from build123d import *

# Parameters (mm, degrees)
SKETCH_1_W          = 90
SKETCH_1_H          = 48
EXTRUDE_1_DEPTH     = 40
CUT_EXTRUDE_1_DEPTH = 40
CUT_EXTRUDE_2_DEPTH = 110.562767398
CUT_EXTRUDE_3_DEPTH = 110.562767398
CUT_EXTRUDE_4_DEPTH = 33
SKETCH_6_W          = 8
SKETCH_6_H          = 40
CUT_EXTRUDE_5_DEPTH = 110.562767398
SKETCH_7_W          = 20
SKETCH_7_H          = 13.155555556
CUT_EXTRUDE_6_DEPTH = 5
SKETCH_8_W          = 28.2
SKETCH_8_H          = 28
EXTRUDE_2_DEPTH     = 3
SKETCH_9_R          = 2.25
EXTRUDE_3_DEPTH     = 4
SKETCH_10_R         = 1.2
CUT_EXTRUDE_7_DEPTH = 104.889364229
FILLET_1_R          = 5
FILLET_2_R          = 2.5


with BuildPart() as part:
    # 스케치1 → 보스-돌출1 (new body)
    with BuildSketch(Plane(origin=(0, 0, 0), x_dir=(0, 0, -1), z_dir=(1, 0, 0))):
        with Locations((45, 24)):
            Rectangle(SKETCH_1_W, SKETCH_1_H)
    extrude(amount=EXTRUDE_1_DEPTH)

    # 스케치2 → 컷-돌출1 (cut)
    with BuildSketch(Plane(origin=(40, 0, 0), x_dir=(0, 0, -1), z_dir=(1, 0, 0))):
        Polygon((79, 44), (83, 44), (83, 38), (85.598076211, 36.5), (83, 35), (83, 33.5), (90, 33.5), (90, 14.5), (83, 14.5), (83, 13), (85.598076211, 11.5), (83, 10), (83, 4), (79, 4), align=None)
        Polygon((0, 38), (63.304035288, 48), (0, 48), align=None)
        Polygon((0, 10), (63.304035288, 0), (0, 0), align=None)
    extrude(amount=-CUT_EXTRUDE_1_DEPTH, mode=Mode.SUBTRACT)

    # 스케치3 → 컷-돌출2 (cut, through all)
    with BuildSketch(Plane(origin=(0, 48, 0), x_dir=(1, 0, 0), z_dir=(0, 1, 0))):
        Polygon((0, 67.846768337), (20, 79), (20, 90), (0, 90), align=None)
    extrude(amount=-CUT_EXTRUDE_2_DEPTH, mode=Mode.SUBTRACT)

    # 스케치4 → 컷-돌출3 (cut, through all)
    with BuildSketch(Plane(origin=(0, 48, 0), x_dir=(1, 0, 0), z_dir=(0, 1, 0))):
        Polygon((40, 63.304035288), (14.807552651, 0), (40, 0), align=None)
    extrude(amount=-CUT_EXTRUDE_3_DEPTH, mode=Mode.SUBTRACT)

    # 스케치5 → 컷-돌출4 (cut)
    with BuildSketch(Plane(origin=(40, 0, 0), x_dir=(0, 0, -1), z_dir=(1, 0, 0))):
        Polygon((4.2, 34.488888889), (63.304035288, 34.488888889), (63.304035288, 48), (0, 38), (0, 10), (63.304035288, 0), (63.304035288, 13.511111111), (4.2, 13.511111111), (4.2, 17.422222222), (63.304035288, 17.422222222), (63.304035288, 30.577777778), (4.2, 30.577777778), align=None)
    extrude(amount=-CUT_EXTRUDE_4_DEPTH, mode=Mode.SUBTRACT)

    # 스케치6 → 컷-돌출5 (cut, through all)
    with BuildSketch(Plane(origin=(40, 0, 0), x_dir=(0, 0, -1), z_dir=(1, 0, 0))):
        with Locations((72, 24)):
            Rectangle(SKETCH_6_W, SKETCH_6_H)
    extrude(amount=-CUT_EXTRUDE_5_DEPTH, mode=Mode.SUBTRACT)

    # 스케치7 → 컷-돌출6 (cut)
    with BuildSketch(Plane.XY.offset(-63.304035288)):
        with Locations((30, 24)):
            Rectangle(SKETCH_7_W, SKETCH_7_H)
    extrude(amount=-CUT_EXTRUDE_6_DEPTH, mode=Mode.SUBTRACT)

    # 스케치8 → 보스-돌출2 (add)
    with BuildSketch(Plane.ZY):
        with Locations((-14.1, 24)):
            Rectangle(SKETCH_8_W, SKETCH_8_H)
    extrude(amount=EXTRUDE_2_DEPTH)

    # 스케치9 → 보스-돌출3 (add)
    with BuildSketch(Plane(origin=(0, 0, -79), x_dir=(-1, 0, 0), z_dir=(0, 0, -1))):
        with Locations(Location((-30, 24, 0), (0, 0, 180))):
            Circle(SKETCH_9_R)
    extrude(amount=EXTRUDE_3_DEPTH)

    # 스케치10 → 컷-돌출7 (cut, through all)
    with BuildSketch(Plane(origin=(0, 0, -83), x_dir=(-1, 0, 0), z_dir=(0, 0, -1))):
        with Locations((-30, 24)):
            Circle(SKETCH_10_R)
    extrude(amount=-CUT_EXTRUDE_7_DEPTH, mode=Mode.SUBTRACT)

    # 필렛1
    # the kernel refuses this fillet: 5 mm, written as the material it takes off along each edge
    with BuildSketch(Plane(origin=(-3, 49.456439237, -28.2), x_dir=(1, 0, 0), z_dir=(0, -1, 0))) as fillet_1_piece_1:
        with BuildLine():
            CenterArc((5, 4.582575695), FILLET_1_R, 180, 66.421821522)
            Line((0, 4.582575695), (-0.1, 4.582575695))
            Line((-0.1, 4.582575695), (-0.1, 0))
            Line((-0.1, 0), (0, -0.1))
            ThreePointArc((0, -0.1), (1.5, -0.1), (2.96, -0.091651514))
            Line((2.96, -0.091651514), (3, 0))
        make_face()
    extrude(amount=50.912878475, mode=Mode.SUBTRACT)
    with BuildSketch(Plane(origin=(16.47898289, 25.901187913, -4.2), x_dir=(0.36975577982440216, 0, -0.9291289809743576), z_dir=(0, -1, 0)), Plane(origin=(16.47898289, 42.96785458, -4.2), x_dir=(0.36975577982440216, 0, -0.9291289809743576), z_dir=(0, -1, 0))) as fillet_1_piece_2:
        with BuildLine():
            CenterArc((FILLET_1_R * 0.67831725528, -FILLET_1_R), FILLET_1_R, 90, 68.299443615)
            Line((-FILLET_1_R * 0.250811725694, -FILLET_1_R * 0.630244220176), (-FILLET_1_R * 0.269394305314, -FILLET_1_R * 0.622849104579))
            Line((-FILLET_1_R * 0.269394305314, -FILLET_1_R * 0.622849104579), (-FILLET_1_R * 0.0135663451056, FILLET_1_R * 0.02))
            Line((-FILLET_1_R * 0.0135663451056, FILLET_1_R * 0.02), (FILLET_1_R * 0.67831725528, FILLET_1_R * 0.02))
            Line((FILLET_1_R * 0.67831725528, FILLET_1_R * 0.02), (FILLET_1_R * 0.67831725528, 0))
        make_face()
    extrude(amount=20.869042493, mode=Mode.SUBTRACT)
    with BuildSketch(Plane(origin=(7.5, 0, -90), x_dir=(0, 0, 1), z_dir=(1, 0, 0))) as fillet_1_piece_3:
        with BuildLine():
            CenterArc((FILLET_1_R, -FILLET_1_R), FILLET_1_R, 90, 90)
            Line((0, -FILLET_1_R), (-FILLET_1_R * 0.02, -FILLET_1_R))
            Line((-FILLET_1_R * 0.02, -FILLET_1_R), (-FILLET_1_R * 0.02, FILLET_1_R * 0.02))
            Line((-FILLET_1_R * 0.02, FILLET_1_R * 0.02), (FILLET_1_R, FILLET_1_R * 0.02))
            Line((FILLET_1_R, FILLET_1_R * 0.02), (FILLET_1_R, 0))
        make_face()
    extrude(amount=45, mode=Mode.SUBTRACT)
    with BuildSketch(Plane(origin=(7.5, 48, -90), x_dir=(0, 0, 1), z_dir=(1, 0, 0))) as fillet_1_piece_4:
        with BuildLine():
            CenterArc((FILLET_1_R, FILLET_1_R), FILLET_1_R, 180, 90)
            Line((0, FILLET_1_R), (-FILLET_1_R * 0.02, FILLET_1_R))
            Line((-FILLET_1_R * 0.02, FILLET_1_R), (-FILLET_1_R * 0.02, -FILLET_1_R * 0.02))
            Line((-FILLET_1_R * 0.02, -FILLET_1_R * 0.02), (FILLET_1_R, -FILLET_1_R * 0.02))
            Line((FILLET_1_R, -FILLET_1_R * 0.02), (FILLET_1_R, 0))
        make_face()
    extrude(amount=45, mode=Mode.SUBTRACT)

    # 필렛2
    fillet_2_edges = [part.edges().sort_by_distance(p)[0] for p in [
        (30, 14.5, -90),
        (30, 33.5, -90),
    ]]
    fillet(fillet_2_edges, radius=FILLET_2_R)


solid = part.part
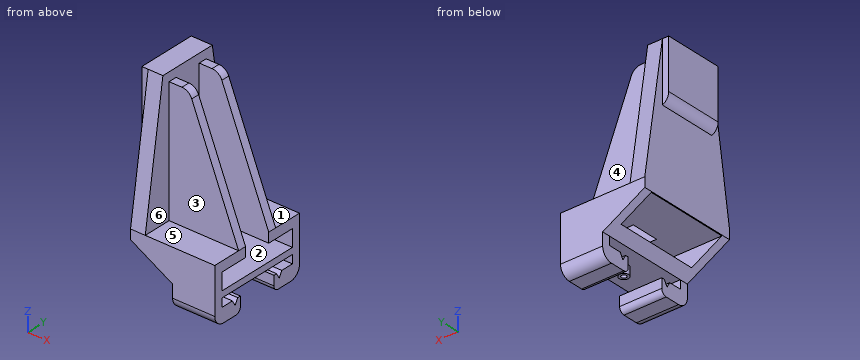
Source: CAD feature listing. Evaluate the final solid. Frame: model axes, mm. Face numbers are marked on the shaded views. A direction names the side the tool comes from. Give positions to 0.01 mm unless a question says otherwise; leave off trailing zeros. Loops run counter-clockwise (first coordinate to the right, second up) from the corner with the lowest first, then second, coordinate; pieces in that order, holes last. Notation, with made-up numbers: (47, 50) -> (87, 50) arc R23 cw to (87, 66) -> close; hole circle Ø7 at (5.5, -31.75). An arc over 180 degrees is marked (long way). Use a Markdown table: item, result. Add a question column.
1) Reachability of the marked faces 4, 5 and 6 from +Z, -Z, +X, -X, +Y, -Y: full face, straight path, thin tool, end or side. Return the list, or none.
2) Section query A-A, the plane y = 24. Return the cut outline in (x, z).
3) Section query C-C, the plane z = -64.5. Return the cut outline in (x, y), then the cut area to 3 significant figures.
4) Pull-direction query (Y, two-part tool) for the marked faces 1, 2 and 3; classes: +Y half, -Y half, draft (parallel to the pull), parting line (faces both ways), or undercut.
5) Line query: line 1 along Y through (x, z) = (30, -81); line 2 along Y through (x, z) = (15.5, -25); line 3 along Y through (x, z) = (29.5, -74.5). Output: solid intervals per line, ascending. Write a range as [from, to].
6) First-contact query: pin 1 (1.5 mm diameter, centred on y = 34.5, z = -25, fed in from -X); pin 2 (5 mm diameter, centred on x = 34.5, y = 15, fed in from -Z); pin 3 (1.5 mm diameter, centred on x = 33, z = -61, fed in from -Y). Flat tips, straight axial feed; report the tip coordinate or a pass-through.
7) Section query B-B, the plane y = 32. Return the cut outline in (x, z).
8) Section query D-D, the plane x = 19. Return the cut outline in (y, z), then the cut area to 3 significant figures.
Numbers:
| question | item | result |
|---|---|---|
| 1 | face 4 | +Z, +X, +Y |
| 1 | face 5 | +Z, +X, -Y |
| 1 | face 6 | +Z, +X |
| 2 | outline | (-3, -23.62) arc R5 ccw to (0, -28.2) -> (0, -67.85) -> (0.27, -68) -> (20, -68) -> (20, -63.3) -> (7, -63.3) -> (7, 0) -> (-3, 0) -> close; (14.62, -76) -> (20, -79) -> (27.75, -79) -> (27.75, -83) -> (28.8, -83) -> (28.8, -76) -> close; (31.2, -83) -> (32.25, -83) -> (32.25, -79) -> (40, -79) -> (40, -76) -> (31.2, -76) -> close |
| 3 | outline | (0, 0) -> (40, 0) -> (40, 17.42) -> (20, 17.42) -> (20, 30.58) -> (40, 30.58) -> (40, 48) -> (0, 48) -> close |
| 3 | area | 1,660 mm2 |
| 4 | face 1 | draft |
| 4 | face 2 | undercut |
| 4 | face 3 | -Y half |
| 5 | line 1 | y = [0, 4], [21.75, 22.8], [25.2, 26.25], [44, 48] |
| 5 | line 2 | y = [13.51, 17.42], [30.58, 34.49] |
| 5 | line 3 | y = [0, 4], [44, 48] |
| 6 | pin 1 | stops at x = -2.96 |
| 6 | pin 2 | stops at z = -89.95 |
| 6 | pin 3 | stops at y = 13.51 |
| 7 | outline | (-3, -23.62) arc R5 ccw to (0, -28.2) -> (0, -67.85) -> (0.27, -68) -> (40, -68) -> (40, -63.3) -> (17.73, -7.35) arc R5 ccw to (13.09, -4.2) -> (7, -4.2) -> (7, 0) -> (-3, 0) -> close; (14.62, -76) -> (20, -79) -> (40, -79) -> (40, -76) -> close |
| 8 | outline | (0, -78.44) -> (48, -78.44) -> (48, -63.3) -> (34.49, -63.3) -> (34.49, -10.53) -> (30.58, -10.53) -> (30.58, -63.3) -> (17.42, -63.3) -> (17.42, -10.53) -> (13.51, -10.53) -> (13.51, -63.3) -> (0, -63.3) -> close; hole (4, -76) -> (44, -76) -> (44, -68) -> (4, -68) -> close |
| 8 | area | 819 mm2 |
